Work out the finished part from the listing and answer in its coordinate system (mm). A direction names the side the tool comes from. Give positions to 0.01 mm unless a question says otherwise; leave off trailing zeros. Write each loop counter-clockwise with the first axis right and the second up, starting at its lowest first coordinate (ties: lowest second). Pieces come first, ordered by that corner, then holes.
1) Determine the mould class of faces 4 (the face through (-1, 1, 56.388)), 5 (the face through (-1, 1, 0)), 6 (the face through (23.56, -40.49, 29.05)) for opening direction X: pulls with the +X half, pulls with the -X half, needs draft (parallel to the pull), parting line crosses it, or undercut.
2) Straight lines are drawn through the part: probe 1 along Z at (x, y) = (10, -23.5); probe 2 along Z at (x, y) = (-24, -8.5); probe 3 along Z at (x, y) = (42.5, 4.5). For each, find the intervals that lie inside material, in ascending order.
3) Find section C-C (x = -9.5). Determine the outline of the cut face in (y, z), plus the area to 3 significant figures.
4) Given pin 1 Ø10 at (x, z) = (-35.5, 25.5) entering from +Y; pin 2 Ø3 at (y, z) = (37, 50) entering from +X; pin 3 Ø20.5 at (x, z) = (5.5, 11.5) entering from +Y, each flat-ended and moving along its own axis, determine where each tip first touches the part or whether it passes through.
5) A tool of negligible diameter and unlimited length cuts with its end or side. For faces 1 (the face through (19.589, -34.515, 60.824)), 2 (the face through (-5, 16.699, 15)), 3 (the face through (-19.589, 34.515, 60.824)), from which of +Z, -Z, +X, -X, +Y, -Y can it reach the whole face along a straight path? Write none if from no direction.
6) Find section B-B (z = 31). Determine the outline of the cut face in (x, y).
7) Find section D-D (y = 0). Determine the outline of the cut face in (x, z).
8) Find section A-A (z = 23.5). Determine the outline of the cut face in (x, y), plus the area to 3 significant figures.
```python
from build123d import *

# Parameters (mm, degrees)
F1_DEPTH  = 56.388
F2_T      = -2.54
F3_W      = 42.9477673024
F3_H      = 39.3949486315
F4_DEPTH  = 25.4
F5_T      = -2.54
F7_DEPTH  = 2.54
F8_R      = 11.4515388828
F9_DEPTH  = 1.27
F11_DEPTH = 1.27


# Not quite as in the source:
# - a shell that OpenCascade refuses in one call is made with other operations: the cavity is built on its own and cut out


with BuildPart() as f1:
    # F0 (on Top) → F1 (new body)
    with BuildSketch(Plane.XY):
        Polygon((46.5280407677, 27.5831491618), (-0.6236875067, 54.0860398741), (-47.1517282744, 26.5028907122), (-46.5280407677, -27.5831491618), (0.6236875067, -54.0860398741), (47.1517282744, -26.5028907122), align=None)
    extrude(amount=F1_DEPTH)

    # F2
    f2_openings = [f1.faces().sort_by_distance(p)[0] for p in [
        (0, 0, 56.388),
    ]]
    offset(amount=F2_T, openings=f2_openings)

    # F3 (on face) → F4 (join)
    with BuildSketch(Plane.XY.offset(2.54)):
        with Locations((-4.2980322614, -2.9984135181)):
            Rectangle(F3_W, F3_H)
    extrude(amount=F4_DEPTH)

    # F5: a shell. OpenCascade refuses it in one call, so the cavity is built on its own and cut out:
    # the body offset inwards by the wall thickness, plus a prism from it out through each open face.
    f5_core = offset(f1.part, amount=F5_T, kind=Kind.INTERSECTION, mode=Mode.PRIVATE)
    f5_exits = [f5_core.faces().sort_by_distance(p)[0] for p in [
        (-4.298032, -2.998414, 25.4),
    ]]
    add(f5_core, mode=Mode.SUBTRACT)
    extrude(f5_exits, amount=-F5_T, mode=Mode.SUBTRACT)

    # F6 (on face) → F7 (join)
    with BuildSketch(Plane.XY.offset(56.388)):
        Polygon((46.5280407677, 27.5831491618), (-0.6236875067, 54.0860398741), (-47.1517282744, 26.5028907122), (-46.5280407677, -27.5831491618), (0.6236875067, -54.0860398741), (47.1517282744, -26.5028907122), align=None)
    extrude(amount=F7_DEPTH)

    # F8 (on face) → F9 (join)
    with BuildSketch(Plane.XY.offset(58.928)):
        Circle(F8_R)
    extrude(amount=F9_DEPTH)

    # F10 (on face) → F11 (join)
    with BuildSketch(Plane.XY.offset(60.198)):
        Polygon((39.6687044392, 22.9401686529), (-0.0324166009, 45.824190106), (-39.7011210401, 22.8840214531), (-39.6687044392, -22.9401686529), (0.0324166009, -45.824190106), (39.7011210401, -22.8840214531), align=None)
    extrude(amount=F11_DEPTH)


solid = f1.part
```
Results:
1. face 4: undercut
1. face 5: needs draft
1. face 6: pulls with the +X half
2. probe 1: z = 0 to 2.54, 56.39 to 58.93, 60.2 to 61.47
2. probe 2: z = 0 to 27.94, 56.39 to 58.93, 60.2 to 61.47
2. probe 3: z = 0 to 2.54, 56.39 to 58.93
3. outline: (-48.4, 0) - (48.82, 0) - (48.82, 58.93) - (6.39, 58.93) - (6.39, 60.2) - (40.35, 60.2) - (40.35, 61.47) - (-40.33, 61.47) - (-40.33, 60.2) - (-6.39, 60.2) - (-6.39, 58.93) - (-48.4, 58.93) - close; hole (-45.48, 2.54) - (-22.7, 2.54) - (-22.7, 27.94) - (-20.16, 27.94) - (-20.16, 2.54) - (14.16, 2.54) - (14.16, 27.94) - (16.7, 27.94) - (16.7, 2.54) - (45.87, 2.54) - (45.87, 56.39) - (-45.48, 56.39) - close
3. area: 1,060 mm2
4. pin 1: stops at y = 36.37
4. pin 2: stops at x = 32.44
4. pin 3: stops at y = 54.09
5. face 1: +Z, +X, -Y
5. face 2: none
5. face 3: +Z, -X, +Y
6. outline: (-47.15, 26.5) - (-46.53, -27.58) - (0.62, -54.09) - (47.15, -26.5) - (46.53, 27.58) - (-0.62, 54.09) - close; hole (-44.59, 25.07) - (-44.01, -26.09) - (0.59, -51.15) - (44.59, -25.07) - (44.01, 26.09) - (-0.59, 51.15) - close
7. outline: (-46.85, 0) - (46.85, 0) - (46.85, 58.93) - (11.45, 58.93) - (11.45, 60.2) - (39.68, 60.2) - (39.68, 61.47) - (-39.68, 61.47) - (-39.68, 60.2) - (-11.45, 60.2) - (-11.45, 58.93) - (-46.85, 58.93) - close; hole (-44.31, 2.54) - (-25.77, 2.54) - (-25.77, 27.94) - (-23.23, 27.94) - (-23.23, 2.54) - (14.64, 2.54) - (14.64, 27.94) - (17.18, 27.94) - (17.18, 2.54) - (44.31, 2.54) - (44.31, 56.39) - (-44.31, 56.39) - close
8. outline: (-47.15, 26.5) - (-46.53, -27.58) - (0.62, -54.09) - (47.15, -26.5) - (46.53, 27.58) - (-0.62, 54.09) - close; (-25.77, -22.7) - (17.18, -22.7) - (17.18, 16.7) - (-25.77, 16.7) - close; hole (-44.59, 25.07) - (-44.01, -26.09) - (0.59, -51.15) - (44.59, -25.07) - (44.01, 26.09) - (-0.59, 51.15) - close; hole (-23.23, -20.16) - (14.64, -20.16) - (14.64, 14.16) - (-23.23, 14.16) - close
8. area: 1,190 mm2
